from build123d import *

# Parameters (mm, degrees)
SKETCH_1_R                = 55
EXTRUDE_1_DEPTH           = 60
EXTRUDE_2_DEPTH           = 60
EXTRUDE_2_DEPTH_BACK      = 58
SKETCH_2_R                = 55
SKETCH_3_R                = 25
CUT_EXTRUDE_1_DEPTH       = 144.349223925
SKETCH_4_R                = 45
CUT_EXTRUDE_2_DEPTH       = 5.5
SKETCH_5_R                = 37.5
CUT_EXTRUDE_3_DEPTH       = 9
SKETCH_8_R                = 50
CUT_EXTRUDE_4_DEPTH       = 93.5
HOLE_WIZARD_1_D           = 3.4
HOLE_WIZARD_1_CBORE_D     = 6
HOLE_WIZARD_1_CBORE_DEPTH = 3.4
PATTERN_CIRCULAR_2_COUNT  = 16
CUT_EXTRUDE_5_DEPTH       = 102.118742081
CUT_EXTRUDE_5_DEPTH_BACK  = 102.118742081
SKETCH_12_R               = 1
CUT_EXTRUDE_6_DEPTH       = 25
SKETCH_13_R               = 1
CUT_EXTRUDE_7_DEPTH       = 48
SKETCH_14_R               = 1
CUT_EXTRUDE_8_DEPTH       = 10
SKETCH_20_R               = 50
CUT_EXTRUDE_15_DEPTH      = 2
SKETCH_18_R               = 42.5
CUT_EXTRUDE_12_DEPTH      = 5
PATTERN_CIRCULAR_3_COUNT  = 12
SKETCH_21_R               = 30
CUT_EXTRUDE_16_DEPTH      = 20
CHAMFER_2_SIZE            = 4


with BuildPart() as part:
    # 草图1 → 凸台-拉伸1 (new body)
    with BuildSketch(Plane.XY):
        Circle(SKETCH_1_R)
    extrude(amount=EXTRUDE_1_DEPTH)

    # 草图2 → 凸台-拉伸2 (add, two sides: drawn at the far end of the back side and taken through both)
    with BuildSketch(Plane(origin=(0, 0, 0), x_dir=(1, 0, 0), z_dir=(0, 1, 0)).offset(-EXTRUDE_2_DEPTH_BACK)):
        with Locations(Location((0, 0, 0), (0, 0, 270))):
            Circle(SKETCH_2_R)
    extrude(amount=EXTRUDE_2_DEPTH + EXTRUDE_2_DEPTH_BACK)

    # 草图3 → 切除-拉伸1 (cut, through all)
    with BuildSketch(Plane.XZ.offset(58)):
        with Locations(Location((0, 0, 0), (0, 0, 270))):
            Circle(SKETCH_3_R)
    extrude(amount=-CUT_EXTRUDE_1_DEPTH, mode=Mode.SUBTRACT)

    # 草图4 → 切除-拉伸2 (cut)
    with BuildSketch(Plane(origin=(0, 60, 0), x_dir=(1, 0, 0), z_dir=(0, 1, 0))):
        with Locations(Location((0, 0, 0), (0, 0, 270))):
            Circle(SKETCH_4_R)
    extrude(amount=-CUT_EXTRUDE_2_DEPTH, mode=Mode.SUBTRACT)

    # 草图5 → 切除-拉伸3 (cut)
    with BuildSketch(Plane(origin=(0, 54.5, 0), x_dir=(1, 0, 0), z_dir=(0, 1, 0))):
        with Locations(Location((0, 0, 0), (0, 0, 270))):
            Circle(SKETCH_5_R)
    extrude(amount=-CUT_EXTRUDE_3_DEPTH, mode=Mode.SUBTRACT)

    # 草图8 → 切除-拉伸4 (cut)
    with BuildSketch(Plane.XZ.offset(58)):
        with Locations(Location((0, 0, 0), (0, 0, 270))):
            Circle(SKETCH_8_R)
    extrude(amount=-CUT_EXTRUDE_4_DEPTH, mode=Mode.SUBTRACT)

    # 打孔尺寸(%根据)内六角圆柱头螺钉的类型1 (through all)
    with Locations(Plane(origin=(0, 35.5, 0), x_dir=(-1, 0, 0), z_dir=(0, -1, 0))):
        with Locations((0, -31)):
            hole_wizard_1 = CounterBoreHole(HOLE_WIZARD_1_D / 2, HOLE_WIZARD_1_CBORE_D / 2, HOLE_WIZARD_1_CBORE_DEPTH)

    # 阵列(圆周)2: 打孔尺寸(%根据)内六角圆柱头螺钉的类型1 ×16 about axis
    pattern_circular_2_axis = Axis((0, 0, 0), (0, 1, 0))
    for i in range(1, PATTERN_CIRCULAR_2_COUNT):
        add(hole_wizard_1.rotate(pattern_circular_2_axis, i * 360 / PATTERN_CIRCULAR_2_COUNT), mode=Mode.SUBTRACT)

    # 草图11 → 切除-拉伸5 (cut, two sides: drawn at the far end of the back side and taken through both)
    with BuildSketch(Plane(origin=(0, 0, 0), x_dir=(0, 0, -1), z_dir=(1, 0, 0)).offset(-CUT_EXTRUDE_5_DEPTH_BACK)):
        Polygon((-55, -58), (55, -58), (55, -17.963274231), align=None)
    extrude(amount=CUT_EXTRUDE_5_DEPTH + CUT_EXTRUDE_5_DEPTH_BACK, mode=Mode.SUBTRACT)

    # 草图12 → 切除-拉伸6 (cut)
    with BuildSketch(Plane(origin=(0, -58, 0), x_dir=(1, 0, 0), z_dir=(0, 1, 0))):
        with Locations(Location((52.5, 0, 0), (0, 0, 270))):
            Circle(SKETCH_12_R)
        with Locations(Location((-52.5, 0, 0), (0, 0, 270))):
            Circle(SKETCH_12_R)
    extrude(amount=CUT_EXTRUDE_6_DEPTH, mode=Mode.SUBTRACT)

    # 草图13 → 切除-拉伸7 (cut)
    with BuildSketch(Plane(origin=(0, -58, 0), x_dir=(1, 0, 0), z_dir=(0, 1, 0))):
        with Locations(Location((0, 52.5, 0), (0, 0, 270))):
            Circle(SKETCH_13_R)
    extrude(amount=CUT_EXTRUDE_7_DEPTH, mode=Mode.SUBTRACT)

    # 草图14 → 切除-拉伸8 (cut)
    with BuildSketch(Plane(origin=(0, -58, 0), x_dir=(1, 0, 0), z_dir=(0, 1, 0))):
        with Locations(Location((0, -52.5, 0), (0, 0, 270))):
            Circle(SKETCH_14_R)
    extrude(amount=CUT_EXTRUDE_8_DEPTH, mode=Mode.SUBTRACT)

    # 草图20 → 切除-拉伸15 (cut)
    with BuildSketch(Plane.XY.offset(60)):
        Circle(SKETCH_20_R)
    extrude(amount=-CUT_EXTRUDE_15_DEPTH, mode=Mode.SUBTRACT)

    # 草图18 → 切除-拉伸12 (cut)
    with BuildSketch(Plane.XY.offset(60)):
        Circle(SKETCH_18_R)
    extrude(amount=-CUT_EXTRUDE_12_DEPTH, mode=Mode.SUBTRACT)

    # 草图16 → M3 螺纹孔2 (revolve, cut)
    with BuildSketch(Plane(origin=(0, 46, 60), x_dir=(0, -1, 0), z_dir=(1, 0, 0))):
        Polygon((0, 0), (0, 8.251075774), (1.25, 7.5), (1.25, 0), align=None)
    hole_wizard_m3_2 = revolve(axis=Axis((0, 46, 66.35), (0, 0, -1)), mode=Mode.SUBTRACT)

    # 阵列(圆周)3: M3 螺纹孔2 ×12 about axis
    pattern_circular_3_axis = Axis((0, 0, 0), (0, 0, 1))
    for i in range(1, PATTERN_CIRCULAR_3_COUNT):
        add(hole_wizard_m3_2.rotate(pattern_circular_3_axis, i * 360 / PATTERN_CIRCULAR_3_COUNT), mode=Mode.SUBTRACT)

    # 草图21 → 切除-拉伸16 (cut)
    with BuildSketch(Plane.XY.offset(55)):
        Circle(SKETCH_21_R)
    extrude(amount=-CUT_EXTRUDE_16_DEPTH, mode=Mode.SUBTRACT)

    # 倒角2
    chamfer_2_edges = [part.edges().sort_by_distance(p)[0] for p in [
        (-55, 0, 60),
    ]]
    chamfer(chamfer_2_edges, length=CHAMFER_2_SIZE)


solid = part.part
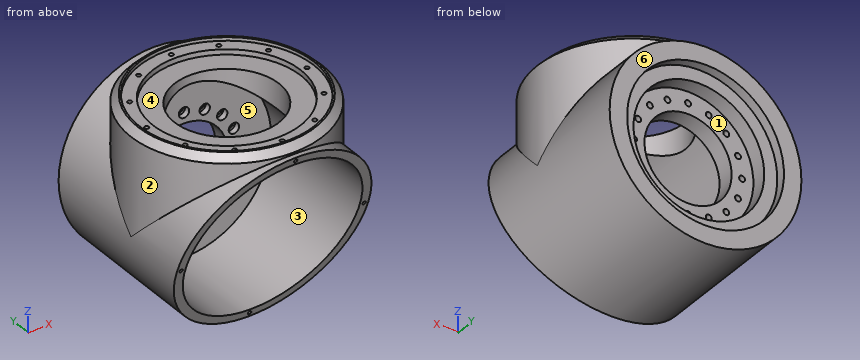
Could you check a few things on this model? Use its own coordinates, in mm. Face numbers are marked on the shaded views. A direction names the side the tool comes from. Give positions to 0.01 mm unless a question says otherwise; leave off trailing zeros. Order: outer loops, then holes, each group sorted by start corner. A loop starts at its lowest first (then second) coordinate and runs counter-clockwise, first axis right, second up.
1. For the marked faces 1, 2 and 3, which set-ups out of +Z, -Z, +X, -X, +Y, -Y let a thin tool reach every point of the face, with its end or its side?
2. Suppose I cut it at B-B (x = -6). Give the number of separate pieces and of enclosed holes in the cut face, plus the area to 3 significant figures.
3. I need wall thicknesses on L1, parallel to X at y = 36, z = 0; L2, parallel to Y at x = 33, z = 26; L3, parallel to X at y = -9, z = 18.5. Which ranges of each line are inside material? Lowest first, please.
4. We'd pull the mould along Y, two halves only. Please class the marked faces 4, 5 and 6: pulls with the +Y half, pulls with the -Y half, needs draft (parallel to the pull), parting line crosses it, or undercut.
5. Suppose I cut it at A-A (z = -5.5). List the corners of the cut face in (x, y) for me.
6. Will these pins go through, and if not, where does the flat tip stop? P1, Ø3, axis at x = -11, z = -26, coming from the +Y side; P2, Ø6.5, axis at x = 32, z = 1.5, coming from the -Y side; P3, Ø3, axis at x = -21.92, z = -21.92, coming from the -Y side; P4, Ø4, axis at x = 23, y = 10, coming from the +Z side.
Solved:
1. face 1: +Y
1. face 2: +Z
1. face 3: -Y
2. separate pieces: 3
2. enclosed holes: 0
2. area: 1,580 mm2
3. L1: x = -55 to -34, -28 to -25, 25 to 28, 34 to 55
3. L2: y = 35.5 to 54.5
3. L3: x = -54.26 to -46.45, 46.45 to 54.26
4. face 4: undercut
4. face 5: pulls with the -Y half
4. face 6: pulls with the +Y half
5. outline: (-54.72, -35.98) - (-49.7, -35.98) - (-49.7, 35.5) - (-24.39, 35.5) - (-24.39, 45.5) - (-37.09, 45.5) - (-37.09, 54.5) - (-44.66, 54.5) - (-44.66, 60) - (-54.72, 60) - close; (24.39, 35.5) - (49.7, 35.5) - (49.7, -35.98) - (54.72, -35.98) - (54.72, 60) - (44.66, 60) - (44.66, 54.5) - (37.09, 54.5) - (37.09, 45.5) - (24.39, 45.5) - close
6. P1: stops at y = 45.5
6. P2: stops at y = 35.5
6. P3: passes through
6. P4: stops at z = -43.3
